Read the model definition and answer for the solid it produces. Units are mm, in the model's axes. A direction names the side the tool comes from. Give positions to 0.01 mm unless a question says otherwise; leave off trailing zeros. Order: outer loops, then holes, each group sorted by start corner. A loop starts at its lowest first (then second) coordinate and runs counter-clockwise, first axis right, second up. Notation, with made-up numbers: (56.25, -28) -> (101.25, -28) arc R12 ccw to (101.25, -23) -> close; hole circle Ø1 at (43.5, -40). An arc over 180 degrees is marked (long way). One line per question, with ' | ' between items. Start each with the question number.
Autodesk Inventor part; units mm, degrees
ref_plane "YZ Plane" through (0, 0, 0) normal (1, 0, 0) x (0, 1, 0)
ref_plane "XZ Plane" through (0, 0, 0) normal (0, 1, 0) x (-1, 0, 0)
ref_plane "XY Plane" through (0, 0, 0) normal (0, 0, 1) x (1, 0, 0)
sketch "Sketch1" plane through (0, 0, 0) normal (0, 1, 0) x (-1, 0, 0)
  line L0 (0, 0) -> (26.304, 0)
  line L1 (26.304, 0) -> (26.304, -38.6)
  line L2 (26.304, -38.6) -> (0, -38.6)
  line L3 (0, -38.6) -> (0, 0)
  dimension "d0" = 38.6
  dimension "d1" = 26.304
extrude "Extrusion1" add sketch "Sketch1" along normal blind 3
sketch "Sketch2" plane through (0, 3, 0) normal (0, 1, 0) x (1, 0, 0)
  line L0 (-19.3893, 5.809) -> (-17.8016, 3.059)
  line L1 (-17.8016, 3.059) -> (-19.3893, 0.309)
  line L2 (-19.3893, 0.309) -> (-22.5647, 0.309)
  line L3 (-22.5647, 0.309) -> (-24.1524, 3.059)
  line L4 (-24.1524, 3.059) -> (-22.5647, 5.809)
  line L5 (-22.5647, 5.809) -> (-19.3893, 5.809)
  line L6 (-19.3893, 38.291) -> (-17.8016, 35.541)
  line L7 (-17.8016, 35.541) -> (-19.3893, 32.791)
  line L8 (-19.3893, 32.791) -> (-22.5647, 32.791)
  line L9 (-22.5647, 32.791) -> (-24.1524, 35.541)
  line L10 (-24.1524, 35.541) -> (-22.5647, 38.291)
  line L11 (-22.5647, 38.291) -> (-19.3893, 38.291)
  line L12 (-3.7393, 5.809) -> (-2.1516, 3.059)
  line L13 (-2.1516, 3.059) -> (-3.7393, 0.309)
  line L14 (-3.7393, 0.309) -> (-6.9147, 0.309)
  line L15 (-6.9147, 0.309) -> (-8.5024, 3.059)
  line L16 (-8.5024, 3.059) -> (-6.9147, 5.809)
  line L17 (-6.9147, 5.809) -> (-3.7393, 5.809)
  line L18 (-3.7393, 38.291) -> (-2.1516, 35.541)
  line L19 (-2.1516, 35.541) -> (-3.7393, 32.791)
  line L20 (-3.7393, 32.791) -> (-6.9147, 32.791)
  line L21 (-6.9147, 32.791) -> (-8.5024, 35.541)
  line L22 (-8.5024, 35.541) -> (-6.9147, 38.291)
  line L23 (-6.9147, 38.291) -> (-3.7393, 38.291)
  line L24 (-26.304, 0) -> (0, 0)
  line L25 (0, 38.6) -> (-26.304, 38.6)
  line L26 (0, 0) -> (0, 38.6)
  point P0 (-20.977, 3.059)
  point P1 (-20.977, 35.541)
  point P2 (-5.327, 3.059)
  point P3 (-5.327, 35.541)
  dimension "d4" = 5.5
  dimension "d6" = 5.5
  dimension "d7" = 5.5
  dimension "d8" = 5.5
  dimension "d9" = 32.482
  dimension "d10" = 32.482
  dimension "d11" = 15.65
  dimension "d12" = 0
  dimension "d13" = 0
  dimension "d14" = 3.059
  dimension "d15" = 5.327
  dimension "d16" = 15.65
extrude "Extrusion2" cut sketch "Sketch2" against normal blind 2.5
sketch "Sketch3" plane through (0, 0, 0) normal (1, 0, 0) x (0, 0, -1)
  line L0 (16.3, 1) -> (17.3, 1)
  line L1 (17.3, 1) -> (17.3, 0)
  line L2 (17.3, 0) -> (16.3, 0)
  line L3 (16.3, 0) -> (16.3, 1)
  line L4 (21.3, 1) -> (22.3, 1)
  line L5 (22.3, 1) -> (22.3, 0)
  line L6 (22.3, 0) -> (21.3, 0)
  line L7 (21.3, 0) -> (21.3, 1)
  line L8 (0, 0) -> (38.6, 0)
  line L9 (0, 0) -> (0, 3)
  dimension "d19" = 1
  dimension "d20" = 1
  dimension "d21" = 1
  dimension "d22" = 4
  dimension "d23" = 16.3
extrude "Extrusion3" cut sketch "Sketch3" against normal blind 24
sketch "Sketch4" plane through (0, 3, 0) normal (0, 1, 0) x (1, 0, 0)
  circle A0 centre (-20.977, 3.059) radius 1.6
  circle A1 centre (-20.977, 35.541) radius 1.6
  circle A2 centre (-5.327, 35.541) radius 1.6
  circle A3 centre (-5.327, 3.059) radius 1.6
  line L0 (-19.3893, 0.309) -> (-22.5647, 0.309)
  line L1 (-3.7393, 0.309) -> (-6.9147, 0.309)
  line L2 (-22.5647, 38.291) -> (-19.3893, 38.291)
  line L3 (-6.9147, 38.291) -> (-3.7393, 38.291)
  line L4 (-24.1524, 3.059) -> (-22.5647, 5.809)
  line L5 (-22.5647, 32.791) -> (-24.1524, 35.541)
  line L6 (-3.7393, 5.809) -> (-2.1516, 3.059)
  line L7 (-3.7393, 38.291) -> (-2.1516, 35.541)
  point P0 (0, 0)
  dimension "d26" = 2.75
  dimension "d27" = 2.75
  dimension "d28" = 2.75
  dimension "d29" = 2.75
  dimension "d30" = 2.75
  dimension "d31" = 2.75
  dimension "d32" = 2.75
  dimension "d33" = 2.75
  dimension "d34" = 3.2
  dimension "d35" = 3.2
  dimension "d36" = 3.2
  dimension "d37" = 3.2
extrude "Extrusion4" cut sketch "Sketch4" against normal through all
sketch "Sketch5" plane through (0, 0, -38.6) normal (0, 0, -1) x (-1, 0, 0)
  line L0 (0, 0) -> (24, 0)
  line L1 (0, 0) -> (26.304, 0)
  line L2 (26.304, 0) -> (26.304, 3)
  line L3 (26.304, 3) -> (0, 3)
  line L4 (0, 3) -> (0, 0)
extrude "Extrusion5" add sketch "Sketch5" along normal blind 2
sketch "Sketch6" plane through (-26.304, 0, 0) normal (0, 0, 1) x (1, 0, 0)
  line L0 (2.304, 0) -> (26.304, 0)
  line L1 (26.304, 0) -> (0, 0)
  line L2 (0, 0) -> (0, 3)
  line L3 (0, 3) -> (26.304, 3)
  line L4 (26.304, 3) -> (26.304, 0)
extrude "Extrusion6" add sketch "Sketch6" along normal blind 2
fillet "Fillet1" radius 4 4 edges at (-26.304, 1.5, -40.6) (0, 1.5, -40.6) (0, 1.5, 2) (-26.304, 1.5, 2)
properties part number "LED_COVER"
Q1. A cutting plane is placed at D-D, the plane x = -3.25. Determine the outline of the cut face in (y, z), then the cut area to 3 significant figures.
Q2. A cutting plane is placed at C-C, the plane x = -15.25. Determine the outline of the cut face in (y, z).
Q3. A cutting plane is placed at B-B, the plane x = -20.75. Determine the outline of the cut face in (y, z).
Q4. Find the intervals of material crossed by line 1 (Z direction, x = -3.75, y = 2.6); line 2 (Z direction, x = -6.75, y = 0.55); line 3 (Z direction, x = -9.5, y = 0.8), in increasing order.
Q5. Determine the mould class of faces 4 (the flat face through (-13, 3, -20)), 5 (the flat face through (-11.8, 0.5, -16.3)), 6 (the flat face through (-13, 2, 2)) for opening direction Z: pulls with the +Z half, pulls with the -Z half, needs draft (parallel to the pull), parting line crosses it, or undercut.
Q6. A cutting plane is placed at A-A, the plane y = 1.65. Give the number of separate pieces and of enclosed holes in the cut face, then the cut area to 3 significant figures.
Q7. Given P1, Ø3, axis at x = -21.5, z = -36, coming from the +Y side; P2, Ø2.5, axis at x = -5.327, z = -3.059, coming from the -Y side, each flat-ended and moving along its own axis, determine where each tip first touches the part or whether it passes through.
Q8. Which of the six approach directions +Z, -Z, +X, -X, +Y, -Y give full straight-line access (tool end or side, diameter ignored) to faces 1 (the cylindrical face through (-1.141, 1.479, 0.797)), 2 (the flat face through (-5, 2, -0.309)), 3 (the flat face through (-12, 1, -17))?
Geometry results:
1) outline: (0, -40.53) -> (3, -40.53) -> (3, -37.44) -> (0.5, -37.44) -> (0.5, -33.64) -> (3, -33.64) -> (3, -4.96) -> (0.5, -4.96) -> (0.5, -1.16) -> (3, -1.16) -> (3, 1.93) -> (0, 1.93) -> (0, -16.3) -> (1, -16.3) -> (1, -17.3) -> (0, -17.3) -> (0, -21.3) -> (1, -21.3) -> (1, -22.3) -> (0, -22.3) -> close | area: 106 mm²
2) outline: (0, -40.6) -> (3, -40.6) -> (3, 2) -> (0, 2) -> (0, -16.3) -> (1, -16.3) -> (1, -17.3) -> (0, -17.3) -> (0, -21.3) -> (1, -21.3) -> (1, -22.3) -> (0, -22.3) -> close
3) outline: (0, -40.6) -> (3, -40.6) -> (3, -38.29) -> (0.5, -38.29) -> (0.5, -37.12) -> (0, -37.12) -> close; (0, -33.96) -> (0.5, -33.96) -> (0.5, -32.79) -> (3, -32.79) -> (3, -5.81) -> (0.5, -5.81) -> (0.5, -4.64) -> (0, -4.64) -> (0, -16.3) -> (1, -16.3) -> (1, -17.3) -> (0, -17.3) -> (0, -21.3) -> (1, -21.3) -> (1, -22.3) -> (0, -22.3) -> close; (0, -1.48) -> (0.5, -1.48) -> (0.5, -0.31) -> (3, -0.31) -> (3, 2) -> (0, 2) -> close
4) line 1: -40.59 to -38.29, -32.79 to -5.81, -0.31 to 1.99 | line 2: -40.6 to -38.29, -32.79 to -22.3, -21.3 to -17.3, -16.3 to -5.81, -0.31 to 2 | line 3: -40.6 to -22.3, -21.3 to -17.3, -16.3 to 2
5) face 4: needs draft | face 5: undercut | face 6: pulls with the +Z half
6) separate pieces: 1 | enclosed holes: 4 | area: 1,000 mm²
7) P1: y = 0.5 | P2: through
8) face 1: +Z, +X, +Y, -Y | face 2: +Y | face 3: +X, -Y
